from build123d import *

# Parameters (mm, degrees)
SKETCH_1_W      = 32
SKETCH_1_H      = 45
SKETCH_1_R      = 1.25
EXTRUDE_1_DEPTH = 1
SKETCH_2_W      = 32
SKETCH_2_H      = 31
EXTRUDE_2_DEPTH = 1.5
SKETCH_3_W      = 32
SKETCH_3_H      = 7
EXTRUDE_3_DEPTH = 1


with BuildPart() as part:
    # 草图1 → 凸台-拉伸1 (new body)
    with BuildSketch(Plane(origin=(0, 0, 0), x_dir=(1, 0, 0), z_dir=(0, 1, 0))):
        with Locations((16, 22.5)):
            Rectangle(SKETCH_1_W, SKETCH_1_H)
        with Locations(Location((30.25, 43.25, 0), (0, 0, 270))):
            Circle(SKETCH_1_R, mode=Mode.SUBTRACT)
        with Locations(Location((30.25, 1.75, 0), (0, 0, 90))):
            Circle(SKETCH_1_R, mode=Mode.SUBTRACT)
        with Locations(Location((1.75, 1.75, 0), (0, 0, 270))):
            Circle(SKETCH_1_R, mode=Mode.SUBTRACT)
        with Locations(Location((1.75, 43.25, 0), (0, 0, 90))):
            Circle(SKETCH_1_R, mode=Mode.SUBTRACT)
    extrude(amount=EXTRUDE_1_DEPTH)

    # 草图2 → 凸台-拉伸2 (add)
    with BuildSketch(Plane(origin=(0, 1, 0), x_dir=(1, 0, 0), z_dir=(0, 1, 0))):
        with Locations((16, 26)):
            Rectangle(SKETCH_2_W, SKETCH_2_H)
    extrude(amount=EXTRUDE_2_DEPTH)

    # 草图3 → 凸台-拉伸3 (add)
    with BuildSketch(Plane(origin=(0, 1, 0), x_dir=(1, 0, 0), z_dir=(0, 1, 0))):
        with Locations((16, 7)):
            Rectangle(SKETCH_3_W, SKETCH_3_H)
    extrude(amount=EXTRUDE_3_DEPTH)


solid = part.part
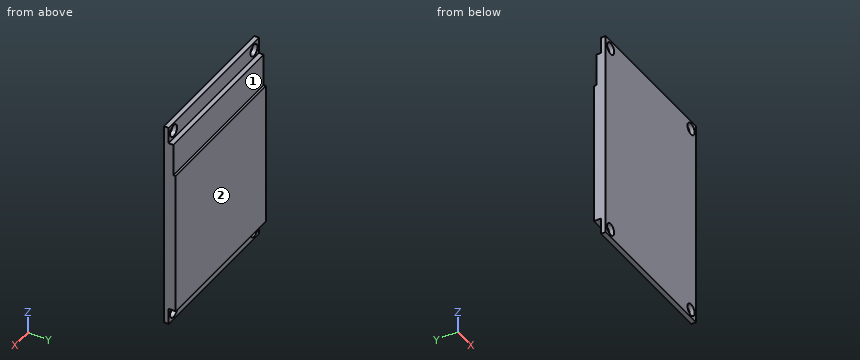
Could you check a few things on this model? Use its own coordinates, in mm. Face numbers are marked on the shaded views. A direction names the side the tool comes from. Give positions to 0.01 mm unless a question says otherwise; leave off trailing zeros. Order: outer loops, then holes, each group sorted by start corner. A loop starts at its lowest first (then second) coordinate and runs counter-clockwise, first axis right, second up.
1. Which directions (+Z, -Z, +X, -X, +Y, -Y) give clear straight access to the entire face, cutting with the end or side of a thin tool? Please do the marked faces 1 and 2.
Answers below:
face 1: +Z, +X, -X, +Y
face 2: +Z, -Z, +X, -X, +Y
2. Suppose I cut it at B-B (z = -43.25). Write out the boundary of the cut face in (x, y).
Answers below:
outline: (0, 0) - (0.5, 0) - (0.5, 1) - (0, 1) - close; (3, 0) - (29, 0) - (29, 1) - (3, 1) - close; (31.5, 0) - (32, 0) - (32, 1) - (31.5, 1) - close
3. Suppose I cut it at A-A (x = 1.75). Write out the boundary of the cut face in (y, z).
Answers below:
outline: (0, -45) - (1, -45) - (1, -44.5) - (0, -44.5) - close; (0, -42) - (1, -42) - (1, -41.5) - (2.5, -41.5) - (2.5, -10.5) - (2, -10.5) - (2, -3.5) - (1, -3.5) - (1, -3) - (0, -3) - close; (0, -0.5) - (1, -0.5) - (1, 0) - (0, 0) - close
4. Suppose I cut it at C-C (x = 11.5). Write out the boundary of the cut face in (y, z).
Answers below:
outline: (0, -45) - (1, -45) - (1, -41.5) - (2.5, -41.5) - (2.5, -10.5) - (2, -10.5) - (2, -3.5) - (1, -3.5) - (1, 0) - (0, 0) - close
5. I need wall thicknesses on L1, parallel to X at y = 0.3, z = -43.25; L2, parallel to Z at x = 26.5, y = 2.15; L3, parallel to Y at x = 18, z = -8. Which ranges of each line are inside material? Lowest first, please.
Answers below:
L1: x = 0 to 0.5, 3 to 29, 31.5 to 32
L2: z = -41.5 to -10.5
L3: y = 0 to 2
6. For pin 1 (3.5 mm diameter, centred on x = 13, z = -6.5, fed in from +Y); pin 2 (1 mm diameter, centred on y = 2, z = -29.5, fed in from -X); pin 3 (3 mm diameter, centred on x = 1.75, z = -43.25, fed in from +Y); pin 4 (1.2 mm diameter, centred on x = 11, y = 2, fed in from -Z), each with a flat end and sliding along its axis, tell me the tip position at first contact or that it passes through.
Answers below:
pin 1: stops at y = 2
pin 2: stops at x = 0
pin 3: stops at y = 1
pin 4: stops at z = -41.5
7. Suppose I cut it at D-D (z = -6). Write out the boundary of the cut face in (x, y), plus the area to 3 significant figures.
Answers below:
outline: (0, 0) - (32, 0) - (32, 2) - (0, 2) - close
area: 64.0 mm2
